The model under review builds one solid part; all positions refer to its coordinate system, in mm. Face numbers are marked on the shaded views. A direction names the side the tool comes from. Round coordinates to 2 decimals unless told otherwise and drop trailing zeros. Order: outer loops, then holes, each group sorted by start corner. A loop starts at its lowest first (then second) coordinate and runs counter-clockwise, first axis right, second up.
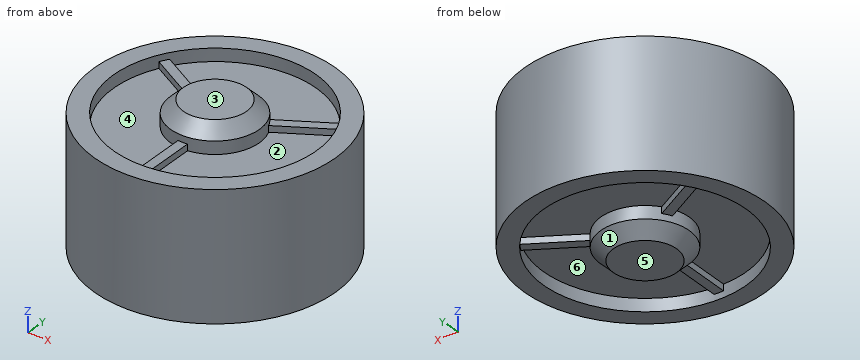
Autodesk Inventor part; units mm, degrees
ref_plane "to_wheel_XY" through (0, 0, 0) normal (0, 0, 1) x (1, 0, 0)
ref_plane "to_wheel_YZ" through (0, 0, 0) normal (1, 0, 0) x (0, 1, 0)
ref_plane "to_wheel_ZX" through (0, 0, 0) normal (0, 1, 0) x (0, 0, 1)
sketch "Sketch_1" plane through (0, 0, 0) normal (1, 0, 0) x (0, 1, 0)
  line L0 (0, -12) -> (0, 12)
  line L1 (0, 12) -> (5, 12)
  line L2 (5, 12) -> (7, 10)
  line L3 (7, 10) -> (7, 8)
  line L4 (7, 8) -> (16, 8)
  line L5 (16, 8) -> (16, 10)
  line L6 (16, 10) -> (19, 10)
  line L7 (19, 10) -> (19, -10)
  line L8 (19, -10) -> (16, -10)
  line L9 (16, -10) -> (16, -8)
  line L10 (16, -8) -> (7, -8)
  line L11 (7, -8) -> (7, -10)
  line L12 (7, -10) -> (5, -12)
  line L13 (5, -12) -> (0, -12)
  line L14 (0, -12) -> (0, 12)
revolve "Revolution1" add sketch "Sketch_1" angle 360 about axis through (0, 0, -12) along (0, 0, -1)
sketch "Sketch_3" plane through (0, 0, 8) normal (0, 0, 1) x (1, 0, 0)
  line L0 (-0.75, -17) -> (0.75, -17)
  line L1 (0.75, -17) -> (0.75, -4)
  line L2 (0.75, -4) -> (-0.75, -4)
  line L3 (-0.75, -4) -> (-0.75, -17)
extrude "Extrusion1" add sketch "Sketch_3" along normal blind 1
sketch "Sketch_2" plane through (0, 0, 8) normal (0, 0, 1) x (1, 0, 0)
  line L0 (3.0891, 2.6495) -> (3.8391, 1.3505)
  line L1 (3.8391, 1.3505) -> (15.0974, 7.8505)
  line L2 (15.0974, 7.8505) -> (14.3474, 9.1495)
  line L3 (14.3474, 9.1495) -> (3.0891, 2.6495)
extrude "Extrusion2" add sketch "Sketch_2" along normal blind 1
sketch "Sketch_4" plane through (0, 0, 8) normal (0, 0, 1) x (1, 0, 0)
  line L0 (-15.0974, 7.8505) -> (-3.8391, 1.3505)
  line L1 (-3.8391, 1.3505) -> (-3.0891, 2.6495)
  line L2 (-3.0891, 2.6495) -> (-14.3474, 9.1495)
  line L3 (-14.3474, 9.1495) -> (-15.0974, 7.8505)
extrude "Extrusion3" add sketch "Sketch_4" along normal blind 1
sketch "Sketch_5" plane through (0, 0, -8) normal (0, 0, 1) x (1, 0, 0)
  line L0 (-0.75, -17) -> (0.75, -17)
  line L1 (0.75, -17) -> (0.75, -4)
  line L2 (0.75, -4) -> (-0.75, -4)
  line L3 (-0.75, -4) -> (-0.75, -17)
extrude "Extrusion4" add sketch "Sketch_5" against normal blind 1
sketch "Sketch_6" plane through (0, 0, -8) normal (0, 0, 1) x (1, 0, 0)
  line L0 (3.0891, 2.6495) -> (3.8391, 1.3505)
  line L1 (3.8391, 1.3505) -> (15.0974, 7.8505)
  line L2 (15.0974, 7.8505) -> (14.3474, 9.1495)
  line L3 (14.3474, 9.1495) -> (3.0891, 2.6495)
extrude "Extrusion5" add sketch "Sketch_6" against normal blind 1
sketch "Sketch_7" plane through (0, 0, -8) normal (0, 0, 1) x (1, 0, 0)
  line L0 (-15.0974, 7.8505) -> (-3.8391, 1.3505)
  line L1 (-3.8391, 1.3505) -> (-3.0891, 2.6495)
  line L2 (-3.0891, 2.6495) -> (-14.3474, 9.1495)
  line L3 (-14.3474, 9.1495) -> (-15.0974, 7.8505)
extrude "Extrusion6" add sketch "Sketch_7" against normal blind 1
ref_plane "to_wheel_XY" through (0, 0, 0) normal (0, 0, 1) x (1, 0, 0)
ref_plane "to_wheel_YZ" through (0, 0, 0) normal (1, 0, 0) x (0, 1, 0)
ref_plane "to_wheel_ZX" through (0, 0, 0) normal (0, 1, 0) x (0, 0, 1)
properties part number "CHAMJ-E50-Rbearing"
(1) Consider section D-D (z = 2.5). Write out the cut boundary in (x, y).
Data:
outline: circle Ø38 at (0, 0)
(2) Draft analysis for pull direction Y (two halves, no side actions). For the marked faces 1, 2 and 3, state which applies: pulls with the +Y half, pulls with the -Y half, needs draft (parallel to the pull), parting line crosses it, or undercut.
Data:
face 1: parting line crosses it
face 2: undercut
face 3: needs draft
(3) Insertion check: pin 1 (1.7 mm diameter, centred on x = -0.5, y = -10.5, fed in from +Z); pin 2 (1.2 mm diameter, centred on x = 0, y = -13.5, fed in from -Z); pin 3 (4.5 mm diameter, centred on x = -9, y = 1.5, fed in from +Z). Each pin has a flat end and moves straight along its axis. Give the tip position at first contact, or say it passes through.
Data:
pin 1: stops at z = 9
pin 2: stops at z = -9
pin 3: stops at z = 10.13
(4) Consider section B-B (x = 0). Write out the cut boundary in (y, z).
Data:
outline: (-19, -10) - (-16, -10) - (-16, -9) - (-7, -9) - (-7, -10) - (-5, -12) - (5, -12) - (7, -10) - (7, -8) - (16, -8) - (16, -10) - (19, -10) - (19, 10) - (16, 10) - (16, 8) - (7, 8) - (7, 10) - (5, 12) - (-5, 12) - (-7, 10) - (-7, 9) - (-16, 9) - (-16, 10) - (-19, 10) - close
(5) Consider section A-A (z = 9.5). Write out the cut boundary in (x, y), and give its area (3 significant figures).
Data:
outline: circle Ø38 at (0, 0); circle Ø14 at (0, 0); hole circle Ø32 at (0, 0)
area: 484 mm2
(6) To check wall thickness, follow probe 1 along X at (y, z) = (0, -8.45); probe 2 along Z at (x, y) = (1, -17); probe 3 along Z at (x, y) = (-15, -3.5). State the ranges of each line that lie inside material, in increasing order.
Data:
probe 1: x = -19 to -16, -7 to 7, 16 to 19
probe 2: z = -10 to 10
probe 3: z = -8 to 8
(7) Consider section C-C (y = 0). Write out the cut boundary in (x, z), and give its area (3 significant figures).
Data:
outline: (-19, -10) - (-16, -10) - (-16, -8) - (-7, -8) - (-7, -10) - (-5, -12) - (5, -12) - (7, -10) - (7, -8) - (16, -8) - (16, -10) - (19, -10) - (19, 10) - (16, 10) - (16, 8) - (7, 8) - (7, 10) - (5, 12) - (-5, 12) - (-7, 10) - (-7, 8) - (-16, 8) - (-16, 10) - (-19, 10) - close
area: 736 mm2
(8) For the marked faces 4, 5 and 6, list the 3-axis set-ups (+Z, -Z, +X, -X, +Y, -Y) from which the entire face can be reached by the end or side of a thin tool; tool diameter is ignored.
Data:
face 4: +Z
face 5: -Z, +X, -X, +Y, -Y
face 6: -Z
